Verification items for the finished model (mm, model axes). A direction names the side the tool comes from. Coordinates: 2 decimals unless noted, no trailing zeros. Order: outer loops, then holes, each group sorted by start corner. A loop starts at its lowest first (then second) coordinate and runs counter-clockwise, first axis right, second up. Notation, with made-up numbers: M 13,36.25 L 70,36.25 A36 cw 70,70.25 Z; hole C 27,18.5 d11. An arc over 180 degrees is marked long. Return JSON: item names as keys, results as strings. Group by question number.
Q1. Mould release check, pull along X, two halves, no side actions. Record for faces 1 (the face through (-10.95, -3.45, -5.4)), 2 (the face through (4.66, -8.96, 9.11)), 3 (the face through (11, -4, -7)): pulls with the +X half, pulls with the -X half, needs draft (parallel to the pull), parting line crosses it, or undercut.
Q2. Thickness scan on probe 1 along Y at (x, z) = (0, 9.4); probe 2 along Z at (x, y) = (-1, -13.75); probe 3 along Y at (x, z) = (0, -9.1). Record the ranges inside material, lowest first.
Q3. Go/stop test with flat-tipped pins: pin 1 Ø8.5 at (x, y) = (-4, -4) entering from +Z; pin 2 Ø4 at (x, z) = (6.5, 6.5) entering from +Y; pin 3 Ø1.5 at (x, z) = (4, -6) entering from -Y; pin 4 Ø9 at (x, y) = (0, 0) entering from +Z. Record where each tip stops, or that it passes through.
Q4. Section check C-C, the plane z = -6. Enter the section's corners in (x, y), then the cut area to 3 significant figures.
Q5. Section check B-B, the plane x = -12. Count the separate pieces of the cut face and the enclosed holes in it, then the cut area to 3 significant figures.
Q6. Section check A-A, the plane z = 0.75. Enter the section's corners in (x, y), then the cut area to 3 significant figures.
Q7. Access from +Z, -Z, +X, -X, +Y, -Y to the whole of each face (thin tool, end or side, straight path). Record for faces 4 (the face through (9.634, 3.034, 3.828)), 5 (the face through (-10.95, -3.45, -8.9)), 6 (the face through (-10.95, -3.45, -1.9)).
from build123d import *

# Parameters (mm, degrees)
SKETCH1_R           = 15
BOSS_EXTRUDE1_DEPTH = 10
SKETCH2_R           = 10.1
CUT_EXTRUDE1_DEPTH  = 24.452078799
SKETCH3_R           = 1.2
SKETCH5_W           = 11
SKETCH5_H           = 3.5
SKETCH7_R           = 0.625
SKETCH9_R           = 11.332657873
BOSS_EXTRUDE2_DEPTH = 9
SKETCH10_R          = 7.5
CUT_EXTRUDE2_DEPTH  = 29.478061732
LPATTERN1_COUNT     = 3
LPATTERN1_PITCH     = 3.5


with BuildPart() as part:
    # Sketch1 → Boss-Extrude1 (new body)
    with BuildSketch(Plane.XY):
        Circle(SKETCH1_R)
    extrude(amount=BOSS_EXTRUDE1_DEPTH)

    # Sketch2 → Cut-Extrude1 (cut, through all)
    with BuildSketch(Plane.XY.offset(10)):
        Circle(SKETCH2_R)
    extrude(amount=-CUT_EXTRUDE1_DEPTH, mode=Mode.SUBTRACT)

    # Sketch3 → Cut-Revolve2 (revolve, cut)
    with BuildSketch(Plane(origin=(0, 0, 0), x_dir=(0, 0, -1), z_dir=(1, 0, 0)), mode=Mode.PRIVATE) as cut_revolve2_sk:
        with Locations((-7, 10.1)):
            Circle(SKETCH3_R)
    revolve(cut_revolve2_sk.sketch.rotate(Axis((0, 0, 0), (0, 0, 1)), 270), axis=Axis((0, 0, 0), (0, 0, 1)), mode=Mode.SUBTRACT)

    # Sketch5 → Revolve1 (revolve)
    with BuildSketch(Plane(origin=(0, 0, 0), x_dir=(0, 0, -1), z_dir=(1, 0, 0)), mode=Mode.PRIVATE) as revolve1_sk:
        with Locations((3.7, -9.35)):
            Rectangle(SKETCH5_W, SKETCH5_H)
    revolve(revolve1_sk.sketch.rotate(Axis((0, 0, 0), (0, 0, 1)), 270), axis=Axis((0, 0, 0), (0, 0, 1)))

    # Sketch7 → Cut-Revolve3 (revolve, cut)
    with BuildSketch(Plane(origin=(0, 0, 0), x_dir=(0, 0, -1), z_dir=(1, 0, 0)), mode=Mode.PRIVATE) as cut_revolve3_sk:
        with Locations((-2.05, 8.85)):
            Circle(SKETCH7_R)
    revolve(cut_revolve3_sk.sketch.rotate(Axis((0, 0, 0), (0, 0, 1)), 90), axis=Axis((0, 0, 0), (0, 0, 1)), mode=Mode.SUBTRACT)

    # Sketch9 → Boss-Extrude2 (add)
    with BuildSketch(Plane(origin=(0, 0, 0), x_dir=(-1, 0, 0), z_dir=(0, 0, -1))):
        with Locations(Location((0, 0, 0), (0, 0, 180))):
            Circle(SKETCH9_R)
    extrude(amount=BOSS_EXTRUDE2_DEPTH)

    # Sketch10 → Cut-Extrude2 (cut, through all)
    with BuildSketch(Plane(origin=(0, 0, -9), x_dir=(-1, 0, 0), z_dir=(0, 0, -1))):
        Circle(SKETCH10_R)
    extrude(amount=-CUT_EXTRUDE2_DEPTH, mode=Mode.SUBTRACT)

    # Sketch11 → Revolve2 (revolve)
    with BuildSketch(Plane(origin=(0, 0, 0), x_dir=(0, 0, -1), z_dir=(1, 0, 0)), mode=Mode.PRIVATE) as revolve2_sk:
        Polygon((9, 11.332657873), (7, 11.332657873), (7, 14.332657873), align=None)
    revolve2 = revolve(revolve2_sk.sketch.rotate(Axis((0, 0, 0), (0, 0, 1)), 90), axis=Axis((0, 0, 0), (0, 0, 1)))

    # LPattern1: Revolve2 ×3
    with Locations(*[(0, 0, i * LPATTERN1_PITCH) for i in range(1, LPATTERN1_COUNT)]):
        add(revolve2)


solid = part.part
Numbers:
{
 "1": {"face 1": "parting line crosses it", "face 2": "undercut", "face 3": "needs draft"},
 "2": {"probe 1": "y = -15 to -10.1, 10.1 to 15", "probe 2": "z = -7.36 to -7, -3.86 to -3.5, -0.36 to 10", "probe 3": "y = -11.1 to -7.6, 7.6 to 11.1"},
 "3": {"pin 1": "stops at z = 1.8", "pin 2": "stops at y = 14.31", "pin 3": "stops at y = -11.03", "pin 4": "passes through"},
 "4": {"outline": "C 0,0 d22.67; hole C 0,0 d15", "area": "227 mm2"},
 "5": {"separate pieces": "3", "enclosed holes": "0", "area": "228 mm2"},
 "6": {"outline": "C 0,0 d30; hole C 0,0 d15.2", "area": "525 mm2"},
 "7": {"face 4": "+Z", "face 5": "-Z", "face 6": "none"}
}
